The model under review builds one solid part; all positions refer to its coordinate system, in mm. Face numbers are marked on the shaded views. A direction names the side the tool comes from. Give positions to 0.01 mm unless a question says otherwise; leave off trailing zeros. Order: outer loops, then holes, each group sorted by start corner. A loop starts at its lowest first (then second) coordinate and runs counter-clockwise, first axis right, second up.
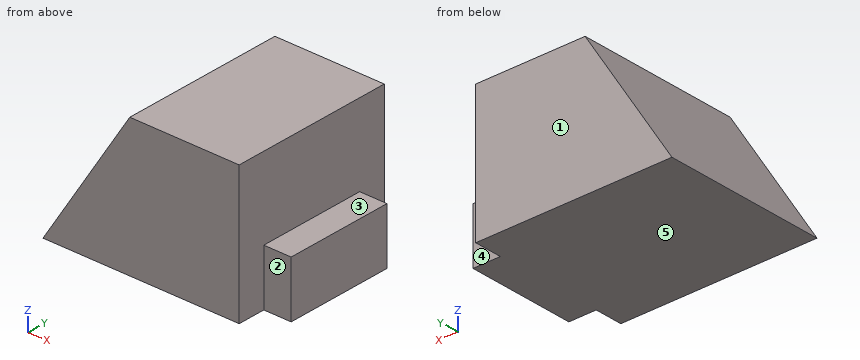
Autodesk Inventor part; units mm, degrees
ref_plane "YZ Plane" through (0, 0, 0) normal (1, 0, 0) x (0, 1, 0)
ref_plane "XZ Plane" through (0, 0, 0) normal (0, 1, 0) x (-1, 0, 0)
ref_plane "XY Plane" through (0, 0, 0) normal (0, 0, 1) x (1, 0, 0)
sketch "Sketch1" plane through (0, 0, 0) normal (0, 0, 1) x (1, 0, 0)
  line L0 (40.3102, 67.1309) -> (91.1102, 67.1309)
  line L1 (91.1102, 67.1309) -> (91.1102, -9.0691)
  line L2 (91.1102, -9.0691) -> (40.3102, -9.0691)
  line L3 (40.3102, -9.0691) -> (40.3102, 67.1309)
  point P0 (0, 0)
  dimension "d0" = 50.8
  dimension "d1" = 76.2
extrude "Extrusion1" add sketch "Sketch1" along normal blind 63.5
sketch "Sketch2" plane through (40.3102, -9.0691, 0) normal (0, -1, 0) x (1, 0, 0)
  line L0 (0, 0) -> (0, 63.5)
  line L1 (50.8, 63.5) -> (0, 63.5)
  line L2 (0, 0) -> (50.8, 0)
  line L3 (0, 0) -> (-40.3102, 0)
  line L4 (0, 63.5) -> (-40.3102, 0)
extrude "Extrusion2" add sketch "Sketch2" against normal blind 76.2
sketch "Sketch6" plane through (91.1102, -9.0691, 0) normal (1, 0, 0) x (0, 0, -1)
  line L0 (-63.5, 0) -> (-63.5, 76.2)
  line L1 (0, 76.2) -> (0, 0)
  line L2 (-25.9302, 38.1) -> (-25.9302, 63.2786)
  line L3 (-25.9302, 63.2786) -> (0, 63.2786)
  line L4 (-25.9302, 38.1) -> (-25.9302, 12.9286)
  line L5 (-25.9302, 38.1) -> (-0.7588, 38.1) construction
  line L6 (-25.9302, 12.9286) -> (0, 12.9286)
  point P0 (0, 9.0691)
  dimension "d11" = 25.1714
  dimension "d12" = 90
  dimension "d13" = 50.35
  dimension "d14" = 25.9302
extrude "Extrusion3" add sketch "Sketch6" along normal blind 12.7
properties part number "mcdave_summo_robot"
1. Take a section at B-B (y = 39.5). Write out the cut boundary in (x, z), and give its area (3 significant figures).
2. Take a section at C-C (x = 97). Write out the cut boundary in (y, z), and give its area (3 significant figures).
3. Take a section at A-A (z = 24.5). Write out the cut boundary in (x, y), and give its area (3 significant figures).
4. For the marked faces 1, 2, 3, 4 and 5, list the 3-axis set-ups (+Z, -Z, +X, -X, +Y, -Y) from which the entire face can be reached by the end or side of a thin tool; tool diameter is ignored.
5. To check wall thickness, follow line 1 (Z direction, x = 98, y = 21.5); line 2 (X direction, y = 18, z = 19.5); line 3 (X direction, y = -1.5, z = 29). State the ranges of each line that lie inside material, in increasing order.
6. Take a section at D-D (z = 7). Write out the cut boundary in (x, y), and give its area (3 significant figures).
7. Insertion check: pin 1 (4 mm diameter, centred on x = 100.5, z = 9.5, fed in from +Y); pin 2 (4 mm diameter, centred on x = 97, z = 7.5, fed in from -Y); pin 3 (4 mm diameter, centred on y = 22.5, z = 49, fed in from -X). Each pin has a flat end and moves straight along its axis. Give the tip position at first contact, or say it passes through.
Answer:
1. outline: (0, 0) - (103.81, 0) - (103.81, 25.93) - (91.11, 25.93) - (91.11, 63.5) - (40.31, 63.5) - close
1. area: 4,830 mm2
2. outline: (3.86, 0) - (54.21, 0) - (54.21, 25.93) - (3.86, 25.93) - close
2. area: 1,310 mm2
3. outline: (15.55, -9.07) - (91.11, -9.07) - (91.11, 3.86) - (103.81, 3.86) - (103.81, 54.21) - (91.11, 54.21) - (91.11, 67.13) - (15.55, 67.13) - close
3. area: 6,400 mm2
4. face 1: +Z, -Z, +X, -X, +Y
4. face 2: +Z, -Z, +X, -Y
4. face 3: +Z, +X, +Y, -Y
4. face 4: +Z, -Z, +X, +Y
4. face 5: -Z, +X, -X, +Y, -Y
5. line 1: z = 0 to 25.93
5. line 2: x = 12.38 to 103.81
5. line 3: x = 18.41 to 91.11
6. outline: (4.44, -9.07) - (91.11, -9.07) - (91.11, 3.86) - (103.81, 3.86) - (103.81, 54.21) - (91.11, 54.21) - (91.11, 67.13) - (4.44, 67.13) - close
6. area: 7,240 mm2
7. pin 1: stops at y = 54.21
7. pin 2: stops at y = 3.86
7. pin 3: stops at x = 29.84
